Here's how the part is built. I have some questions about the finished solid (model axes, mm). A direction names the side the tool comes from. Coordinates: 2 decimals unless noted, no trailing zeros. Write each loop counter-clockwise with the first axis right and the second up, starting at its lowest first coordinate (ties: lowest second). Pieces come first, ordered by that corner, then holes.
Autodesk Inventor part; units mm, degrees
ref_plane "YZ Plane" through (0, 0, 0) normal (1, 0, 0) x (0, 1, 0)
ref_plane "XZ Plane" through (0, 0, 0) normal (0, 1, 0) x (-1, 0, 0)
ref_plane "XY Plane" through (0, 0, 0) normal (0, 0, 1) x (1, 0, 0)
sketch "Szkic1" plane through (0, 0, 0) normal (0, 0, 1) x (1, 0, 0)
  line L0 (24.72, -24.72) -> (24.72, -14.42)
  line L1 (25.2197, -24.72) -> (24.72, -24.72)
  line L2 (24.72, -14.42) -> (25.2197, -14.42)
  line L3 (0, -39.14) -> (10.3, -39.14)
  line L4 (-14.42, -14.42) -> (-14.42, -24.72)
  line L5 (10.3, 0) -> (0, 0)
  line L6 (10.225, -25.645) -> (10.225, -13.495)
  line L7 (10.225, -25.645) -> (0.075, -25.645)
  line L8 (0.075, -13.495) -> (0.075, -25.645)
  line L9 (0.075, -13.495) -> (10.225, -13.495)
  line L10 (-14.9619, -24.72) -> (-14.9619, -24.7024)
  arc A0 (-14.9619, -24.7024) -> (0.075, -39.676) centre (5.1314, -19.5612) ccw
  arc A1 (10.3, -39.6475) -> (25.2201, -24.72) centre (5.1314, -19.5612) ccw
  line L11 (-14.9619, -14.42) -> (-14.42, -14.42)
  line L12 (24.72, -14.42) -> (25.2247, -14.42)
  line L13 (-14.42, -24.72) -> (-14.9619, -24.72)
  line L14 (0.075, -39.14) -> (0.075, -39.676)
  line L15 (0.075, 0.5536) -> (0.075, 0)
  line L16 (0.075, -13.495) -> (0.075, -25.645)
  line L17 (10.3, -39.6475) -> (10.3, -39.14)
  line L18 (10.3, 0) -> (10.3, 0.5251)
  line L19 (25.2201, -24.72) -> (24.72, -24.72)
  arc A2 (25.2247, -14.42) -> (10.3, 0.5251) centre (5.1314, -19.5612) ccw
  arc A3 (0.075, 0.5536) -> (-14.9619, -14.42) centre (5.1314, -19.5612) ccw
  circle A4 centre (5.1581, -35.1055) radius 1.75
  circle A5 centre (16.1418, -30.5337) radius 1.75
  circle A6 centre (20.6757, -19.5344) radius 1.75
  circle A7 centre (16.1039, -8.5508) radius 1.75
  circle A8 centre (5.1046, -4.0169) radius 1.75
  circle A9 centre (-5.879, -8.5887) radius 1.75
  circle A10 centre (-10.4129, -19.588) radius 1.75
  circle A11 centre (-5.8412, -30.5716) radius 1.75
  point P0 (5.15, -19.57)
  point P1 (-14.9574, -24.72)
  dimension "d0" = 3.5
  dimension "d3" = 360
extrude "Wyciągnięcie proste1" add sketch "Szkic1" along normal blind 9.7 contours L1 A1 L17 L3 L14 A0 L13 L4 L11 A3 L15 L5 L18 A2 L12 L2 L0
sketch "Szkic2" plane through (0, 0, 0) normal (0, 0, -1) x (-1, 0, 0)
  circle A0 centre (-16.1039, -8.5508) radius 1.75
  circle A1 centre (-16.1039, -8.5508) radius 3
  arc A2 (-10.3, 0.5251) -> (-25.2247, -14.42) centre (-5.1314, -19.5612) ccw
  arc A3 (-0.075, -39.676) -> (14.9574, -24.72) centre (-5.1314, -19.5612) ccw
  circle A4 centre (-16.1418, -30.5337) radius 3
  circle A5 centre (5.8412, -30.5716) radius 3
  circle A6 centre (5.879, -8.5887) radius 3
  point P0 (0, 0)
  dimension "d7" = 6
  dimension "d10" = 360
extrude "Wyciągnięcie proste2" cut sketch "Szkic2" against normal blind 3.7
sketch "Szkic3" plane through (0, 0, 0) normal (0, 0, -1) x (-1, 0, 0)
  circle A0 centre (5.8412, -30.5716) radius 3
  circle A1 centre (5.879, -8.5887) radius 3
  circle A2 centre (-16.1418, -30.5337) radius 3
  circle A3 centre (-16.1039, -8.5508) radius 3
  line L0 (-24.72, -14.42) -> (-25.2247, -14.42)
  line L1 (-24.72, -24.72) -> (-24.72, -14.42)
  line L2 (-25.2201, -24.72) -> (-24.72, -24.72)
  arc A4 (-25.2201, -24.72) -> (-10.3, -39.6475) centre (-5.1314, -19.5612) ccw
  line L3 (-10.3, -39.14) -> (-10.3, -39.6475)
  line L4 (-0.075, -39.14) -> (-10.3, -39.14)
  line L5 (-0.075, -39.676) -> (-0.075, -39.14)
  arc A5 (-0.075, -39.676) -> (14.9574, -24.72) centre (-5.1314, -19.5612) ccw
  line L6 (14.42, -24.72) -> (14.9574, -24.72)
  line L7 (14.42, -14.42) -> (14.42, -24.72)
  line L8 (14.9619, -14.42) -> (14.42, -14.42)
  arc A6 (14.9619, -14.42) -> (-0.075, 0.5536) centre (-5.1314, -19.5612) ccw
  line L9 (-0.075, 0) -> (-0.075, 0.5536)
  line L10 (-10.3, 0) -> (-0.075, 0)
  line L11 (-10.3, 0.5251) -> (-10.3, 0)
  arc A7 (-10.3, 0.5251) -> (-25.2247, -14.42) centre (-5.1314, -19.5612) ccw
  circle A8 centre (10.4129, -19.588) radius 1.75
  circle A9 centre (-5.1581, -35.1055) radius 1.75
  circle A10 centre (-20.6757, -19.5344) radius 1.75
  circle A11 centre (-5.1046, -4.0169) radius 1.75
  line L12 (-10.225, -25.645) -> (-0.075, -25.645)
  line L13 (-10.225, -13.495) -> (-10.225, -25.645)
  line L14 (-0.075, -13.495) -> (-10.225, -13.495)
  line L15 (-0.075, -25.645) -> (-0.075, -13.495)
  line L16 (-10.225, -13.495) -> (-8.225, -13.495)
  line L17 (-8.225, -13.495) -> (-8.225, -25.645)
  line L18 (-8.225, -25.645) -> (-10.225, -25.645)
  line L19 (-10.225, -25.645) -> (-10.225, -13.495)
  line L20 (-0.075, -25.645) -> (-2.075, -25.645)
  line L21 (-2.075, -25.645) -> (-2.075, -13.495)
  line L22 (-2.075, -13.495) -> (-0.075, -13.495)
  line L23 (-0.075, -13.495) -> (-0.075, -25.645)
  point P0 (0, 0)
  dimension "d14" = 2
  dimension "d15" = 2
extrude "Wyciągnięcie proste3" add sketch "Szkic3" against normal blind 4.7 contours L13 L14 L17 L12 | L21 L14 L15 L12
sketch "Szkic4" plane through (0, 0, 9.7) normal (0, 0, 1) x (1, 0, 0)
  line L0 (24.72, -14.42) -> (25.2247, -14.42)
  arc A0 (25.2247, -14.42) -> (10.3, 0.5251) centre (5.1314, -19.5612) ccw
  line L1 (10.3, 0.5251) -> (10.3, 0)
  line L2 (10.3, 0) -> (0.075, 0)
  line L3 (0.075, 0) -> (0.075, 0.5536)
  arc A1 (0.075, 0.5536) -> (-14.9619, -14.42) centre (5.1314, -19.5612) ccw
  line L4 (-14.9619, -14.42) -> (-14.42, -14.42)
  line L5 (-14.42, -14.42) -> (-14.42, -24.72)
  line L6 (-14.42, -24.72) -> (-14.9574, -24.72)
  arc A2 (-14.9574, -24.72) -> (0.075, -39.676) centre (5.1314, -19.5612) ccw
  line L7 (0.075, -39.676) -> (0.075, -39.14)
  line L8 (0.075, -39.14) -> (10.3, -39.14)
  line L9 (10.3, -39.14) -> (10.3, -39.6475)
  arc A3 (10.3, -39.6475) -> (25.2201, -24.72) centre (5.1314, -19.5612) ccw
  line L10 (25.2201, -24.72) -> (24.72, -24.72)
  line L11 (24.72, -24.72) -> (24.72, -14.42)
  circle A4 centre (-10.4129, -19.588) radius 1.75
  circle A5 centre (5.1581, -35.1055) radius 1.75
  circle A6 centre (20.6757, -19.5344) radius 1.75
  circle A7 centre (5.1046, -4.0169) radius 1.75
  circle A8 centre (-5.8412, -30.5716) radius 1.75
  circle A9 centre (-5.879, -8.5887) radius 1.75
  circle A10 centre (16.1039, -8.5508) radius 1.75
  circle A11 centre (16.1418, -30.5337) radius 1.75
  line L12 (10.225, -25.645) -> (0.075, -25.645)
  line L13 (0.075, -25.645) -> (0.075, -13.495)
  line L14 (0.075, -13.495) -> (10.225, -13.495)
  line L15 (10.225, -13.495) -> (10.225, -25.645)
  line L16 (10.3, 0.5251) -> (10.3, 0)
  line L17 (10.3, 0.5251) -> (0.075, 0.5536)
  line L18 (10.3, 0) -> (0.075, 0)
  circle A12 centre (5.1314, -19.5612) radius 20.2325
  point P0 (0, 0)
  point P1 (-14.4371, -14.42)
  point P2 (0.075, 0.0293)
  point P3 (0.075, -39.1517)
  point P4 (-14.4324, -24.72)
  point P5 (24.72, -24.6249)
  point P6 (10.2329, -39.14)
  point P7 (24.72, -14.4975)
extrude "Wyciągnięcie proste4" cut sketch "Szkic4" against normal through all contours L11 A12 L1 A0 L0 | L11 L10 A3 L9 L8 A12 | L7 A2 L6 A12 | A12 L4 A1 L3
sketch "Szkic5" plane through (0, 0, 0) normal (0, 0, -1) x (-1, 0, 0)
  line L0 (-10.225, -13.495) -> (-10.225, -25.645)
  line L1 (-8.225, -13.495) -> (-10.225, -13.495)
  line L2 (-2.075, -13.495) -> (-8.225, -13.495)
  line L3 (-0.075, -13.495) -> (-2.075, -13.495)
  line L4 (-0.075, -25.645) -> (-0.075, -13.495)
  line L5 (-2.075, -25.645) -> (-0.075, -25.645)
  line L6 (-8.225, -25.645) -> (-2.075, -25.645)
  line L7 (-10.225, -25.645) -> (-8.225, -25.645)
  line L8 (-10.2317, -25.6607) -> (-10.2317, -13.4607)
  line L9 (-0.0317, -13.4607) -> (-10.2317, -13.4607)
  circle A0 centre (-5.1314, -15.0608) radius 0.8097
  line L10 (-0.0317, -25.6607) -> (-0.0317, -13.4607)
  line L11 (-10.2317, -25.6607) -> (-0.0317, -25.6607)
  circle A1 centre (-5.1314, -19.5612) radius 3.4994
  circle A2 centre (-5.1314, -24.061) radius 0.8096
  arc A3 (-10.3, 0) -> (-24.72, -14.4975) centre (-5.1314, -19.5612) ccw
  point P0 (0, 0)
  point P1 (-5.1317, -19.5607)
extrude "Wyciągnięcie proste5" cut sketch "Szkic5" against normal through all contours L1 L2 L3 L4 L5 L6 L7 L0 | A1
extrude "Wyciągnięcie proste6" add sketch "Szkic5" against normal blind 7.3 contours L1 L2 L3 L4 L5 L6 L7 L0
sketch "Szkic6" plane through (0, 0, 0) normal (0, 0, -1) x (-1, 0, 0)
  arc A0 (-10.3, 0) -> (-24.72, -14.4975) centre (-5.1314, -19.5612) ccw
  circle A1 centre (-5.1314, -19.5612) radius 3.4994
  circle A2 centre (-5.1314, -19.5612) radius 20.5
  circle A3 centre (-5.1314, -24.061) radius 0.8096
  circle A4 centre (-5.1314, -19.5612) radius 3.4994
  circle A5 centre (-5.1314, -15.0608) radius 0.8097
  circle A6 centre (-5.1046, -4.0169) radius 1.75
  circle A7 centre (-20.6757, -19.5344) radius 1.75
  circle A8 centre (-5.1581, -35.1055) radius 1.75
  circle A9 centre (10.4129, -19.588) radius 1.75
  circle A10 centre (-16.1039, -8.5508) radius 3
  circle A11 centre (-16.1418, -30.5337) radius 3
  circle A12 centre (5.879, -8.5887) radius 3
  circle A13 centre (5.8412, -30.5716) radius 3
  arc A14 (-0.075, -39.1517) -> (14.4324, -24.72) centre (-5.1314, -19.5612) ccw
  line L0 (14.42, -24.72) -> (14.4324, -24.72)
  line L1 (14.42, -14.42) -> (14.42, -24.72)
  line L2 (14.4371, -14.42) -> (14.42, -14.42)
  arc A15 (14.4371, -14.42) -> (-0.075, 0.0293) centre (-5.1314, -19.5612) ccw
  line L3 (-0.075, 0) -> (-0.075, 0.0293)
  line L4 (-10.3, 0) -> (-0.075, 0)
  arc A16 (-10.3, 0) -> (-24.72, -14.4975) centre (-5.1314, -19.5612) ccw
  line L5 (-24.72, -24.6249) -> (-24.72, -14.4975)
  arc A17 (-24.72, -24.6249) -> (-10.2329, -39.14) centre (-5.1314, -19.5612) ccw
  line L6 (-0.075, -39.14) -> (-10.2329, -39.14)
  line L7 (-0.075, -39.1517) -> (-0.075, -39.14)
  line L8 (-24.72, -6.5254) -> (-24.72, -33.3555)
  line L9 (14.4371, -5.2931) -> (14.4371, -36.8555)
  line L10 (-20.6757, -39.1517) -> (13.3882, -39.1517)
  line L11 (-24, 0) -> (14, 0)
  point P0 (0, 0)
  point P1 (-24.72, -25.6056)
  point P2 (-11.1697, -39.1517)
  point P3 (-0.075, -39.1517)
  point P4 (-0.075, -39.1517)
  point P5 (0.907, -39.1517)
  point P6 (14.4371, -25.6707)
  point P7 (1.0013, 0)
  point P8 (0.0373, 0)
  point P9 (14.4371, -13.4517)
  point P10 (-11.264, 0)
  point P11 (-24.72, -13.5168)
  dimension "d24" = 41
extrude "Wyciągnięcie proste7" add sketch "Szkic6" against normal up to surface (9.7 mm away) contours A0 L8 A2 L11 | A17 L6 L7 L10 A2 L8 | L11 A2 L9 A15 | L9 A2 L10 A14 L0 L1 L2
sketch "Szkic7" plane through (0, 0, 9.7) normal (0, 0, 1) x (1, 0, 0)
  line L0 (10.225, -25.645) -> (0.075, -25.645)
  line L1 (0.075, -25.645) -> (0.075, -13.495)
  line L2 (0.075, -13.495) -> (10.225, -13.495)
  line L3 (10.225, -13.495) -> (10.225, -25.645)
  circle A0 centre (16.1418, -30.5337) radius 1.75
  circle A1 centre (16.1039, -8.5508) radius 1.75
  circle A2 centre (-5.879, -8.5887) radius 1.75
  circle A3 centre (-5.8412, -30.5716) radius 1.75
  circle A4 centre (5.1046, -4.0169) radius 1.75
  circle A5 centre (20.6757, -19.5344) radius 1.75
  circle A6 centre (5.1581, -35.1055) radius 1.75
  circle A7 centre (-10.4129, -19.588) radius 1.75
  line L4 (24.72, -13.5168) -> (24.72, -25.6056)
  arc A8 (24.72, -13.5168) -> (11.264, 0) centre (5.1314, -19.5612) ccw
  line L5 (0.075, 0) -> (11.264, 0)
  line L6 (0.075, 0) -> (0.075, 0.0293)
  arc A9 (0.075, 0.0293) -> (-0.0373, 0) centre (5.1314, -19.5612) ccw
  line L7 (-1.0013, 0) -> (-0.0373, 0)
  arc A10 (-1.0013, 0) -> (-14.4371, -13.4517) centre (5.1314, -19.5612) ccw
  line L8 (-14.4371, -25.6707) -> (-14.4371, -13.4517)
  arc A11 (-14.4371, -25.6707) -> (-0.907, -39.1517) centre (5.1314, -19.5612) ccw
  line L9 (11.1697, -39.1517) -> (-0.907, -39.1517)
  arc A12 (11.1697, -39.1517) -> (24.72, -25.6056) centre (5.1314, -19.5612) ccw
  line L10 (0.075, 0) -> (-0.0373, 0)
  point P0 (0, 0)
extrude "Wyciągnięcie proste8" cut sketch "Szkic7" against normal through all contours L10 A9 L6
sketch "Szkic8" plane through (0, 0, 7.3) normal (0, 0, 1) x (1, 0, 0)
  line L0 (10.225, -25.645) -> (0.075, -25.645)
  line L1 (10.225, -13.495) -> (10.225, -25.645)
  line L2 (0.075, -13.495) -> (10.225, -13.495)
  line L3 (0.075, -25.645) -> (0.075, -13.495)
  circle A0 centre (5.1314, -15.0608) radius 0.8097
  circle A1 centre (5.1314, -19.5612) radius 3.4994
  circle A2 centre (5.1314, -24.061) radius 0.8096
  point P0 (0, 0)
extrude "Wyciągnięcie proste9" cut sketch "Szkic8" against normal blind 4
sketch "Szkic9" plane through (0, 0, 0) normal (0, 0, -1) x (-1, 0, 0)
  circle A0 centre (-5.1314, -15.0608) radius 0.8097
  circle A1 centre (-5.1314, -24.061) radius 0.8096
  point P0 (0, 0)
extrude "Wyciągnięcie proste10" add sketch "Szkic9" against normal up to surface (3.3 mm away)
sketch "Szkic10" plane through (0, 0, 9.7) normal (0, 0, 1) x (1, 0, 0)
  line L0 (0.075, -25.645) -> (0.075, -13.495)
  line L1 (10.225, -25.645) -> (0.075, -25.645)
  line L2 (10.225, -13.495) -> (10.225, -25.645)
  line L3 (0.075, -13.495) -> (10.225, -13.495)
  line L4 (10.725, -26.145) -> (-0.425, -26.145)
  line L5 (-0.425, -26.145) -> (-0.425, -12.995)
  line L6 (-0.425, -12.995) -> (10.725, -12.995)
  line L7 (10.725, -12.995) -> (10.725, -26.145)
  point P0 (0, 0)
  dimension "d33" = 0.5
extrude "Wyciągnięcie proste11" cut sketch "Szkic10" against normal up to surface (6.4 mm away) contours L0 L3 L2 L1 | L4 L5 L6 L7
properties part number "GripperBaseCircularUpper"
1) Imagine slicing it at A-A on x = 16. Please give me the cut outline in (y, z), then the cut area to 3 significant figures.
Values follow:
outline: (-36.94, 0) - (-33.53, 0) - (-33.53, 3.7) - (-32.28, 3.7) - (-32.28, 9.7) - (-36.94, 9.7) - close; (-28.79, 3.7) - (-27.54, 3.7) - (-27.54, 0) - (-11.55, 0) - (-11.55, 3.7) - (-10.3, 3.7) - (-10.3, 9.7) - (-28.79, 9.7) - close; (-6.8, 3.7) - (-5.55, 3.7) - (-5.55, 0) - (-2.18, 0) - (-2.18, 9.7) - (-6.8, 9.7) - close
area: 251 mm2
2) Imagine slicing it at B-B on z = 2.5. Count the separate pieces of the cut face and the enclosed holes in it, then the cut area to 3 significant figures.
Values follow:
separate pieces: 1
enclosed holes: 9
area: 1,100 mm2
3) Imagine slicing it at C-C on y = -34.5. Please give me the cut outline in (x, z), then the cut area to 3 significant figures.
Values follow:
outline: (-8.91, 0) - (3.52, 0) - (3.52, 9.7) - (-8.91, 9.7) - close; (6.8, 0) - (19.17, 0) - (19.17, 9.7) - (6.8, 9.7) - close
area: 240 mm2
4) We'd pull the mould along X, two halves only. Please class faces 4 (the face through (5, -11, 9.7)), 5 (the face through (-14.437, -19, 5)), 6 (the face through (-5.071, -7.036, 6.658)): pulls with the +X half, pulls with the -X half, needs draft (parallel to the pull), parting line crosses it, or undercut.
Values follow:
face 4: needs draft
face 5: pulls with the -X half
face 6: undercut
5) I need wall thicknesses on probe 1 along Y at (x, z) = (8.5, 6.75) (3 decimals); probe 2 along Y at (x, z) = (-7, 0.5); probe 3 along X at (y, z) = (-6, 3.25). Which ranges of each line are inside material? Lowest first, please.
Values follow:
probe 1: y = -39.152 to -26.145, -12.995 to 0
probe 2: y = -36.09 to -33.34, -27.8 to -11.37, -5.81 to -3.04
probe 3: x = -10.24 to -7.4, -4.36 to 14.52, 17.68 to 20.5
6) Imagine slicing it at D-D on y = -3.5. Please give me the cut outline in (x, z), then the cut area to 3 significant figures.
Values follow:
outline: (-7.61, 0) - (3.43, 0) - (3.43, 9.7) - (-7.61, 9.7) - close; (6.78, 0) - (17.87, 0) - (17.87, 9.7) - (6.78, 9.7) - close
area: 215 mm2
7) Will these pins go through, and if not, where does the flat tip stop? pin 1 (3 mm diameter, centred on x = 16.1, y = -8.55, fed in from +Z); pin 2 (9.5 mm diameter, centred on x = -5.88, y = -8.59, fed in from -Z); pin 3 (5 mm diameter, centred on x = 16, z = 7, fed in from -Y); pin 4 (3 mm diameter, centred on x = -5.5, y = -8, fed in from -Z).
Values follow:
pin 1: passes through
pin 2: stops at z = 0
pin 3: stops at y = -38.28
pin 4: stops at z = 3.7
8) On a 3-axis mill with a long thin cutter (end or side, diameter ignored), from which of +Z, -Z, +X, -X, +Y, -Y can I reach the whole of each face in a straight line? I mean faces 1 (the face through (5, -12.995, 7)), 2 (the face through (-8, -31, 3.7)), 3 (the face through (3.815, -5.2, 4.782)). Say none if no direction works.
Values follow:
face 1: +Z
face 2: -Z
face 3: +Z, -Z
